Can you work these out from the drawing? Everything is in mm from the part's minimum corner. A direction names the side the tool comes from. Round coordinates to 2 decimals unless told otherwise and drop trailing zeros. Write each loop counter-clockwise with the first axis right and the second up, starting at its lowest first coordinate (ties: lowest second). Pieces come first, ordered by that corner, then holes. Notation, with made-up numbers: M 63.25,30 L 71.25,30 A15 ccw 71.25,35 Z; hole C -13.75,11 d9. An arc over 180 degrees is marked long. Answer in a Markdown table with one row per item. Add a question column.
(1) If I drill on probe 1 along Y at (x, z) = (10.5, 9.75); probe 2 along Z at (x, y) = (15, 16); probe 3 along Y at (x, z) = (10.5, 20), over which ranges is the centre line in solid material (lowest first)?
(2) Suppose I cut it at D-D, the plane y = 14.75. Write out the boundary of the cut face in (x, z).
(3) Suppose I cut it at A-A, the plane x = 10.5. Write out the boundary of the cut face in (y, z).
(4) For the marked faces 1 and 2, which set-ups out of +Z, -Z, +X, -X, +Y, -Y let a thin tool reach every point of the face, with its end or its side?
(5) Suppose I cut it at B-B, the plane y = 8.5. Write out the boundary of the cut face in (x, z), then the cut area to 3 significant figures.
(6) I'm going to push flat-ended pins straight in: pin 1 (12 mm diameter, centred on x = 9.5, y = 11, fed in from -Z); pin 2 (3 mm diameter, centred on x = 15, z = 4.5, fed in from +Y); pin 3 (2 mm diameter, centred on x = 4.5, z = 23, fed in from -Y); pin 4 (6 mm diameter, centred on y = 15, z = 6.5, fed in from +X). Where does each tip first touch, or does it pass through?
(7) Suppose I cut it at C-C, the plane z = 14.75. Write out the boundary of the cut face in (x, y), then the cut area to 3 significant figures.
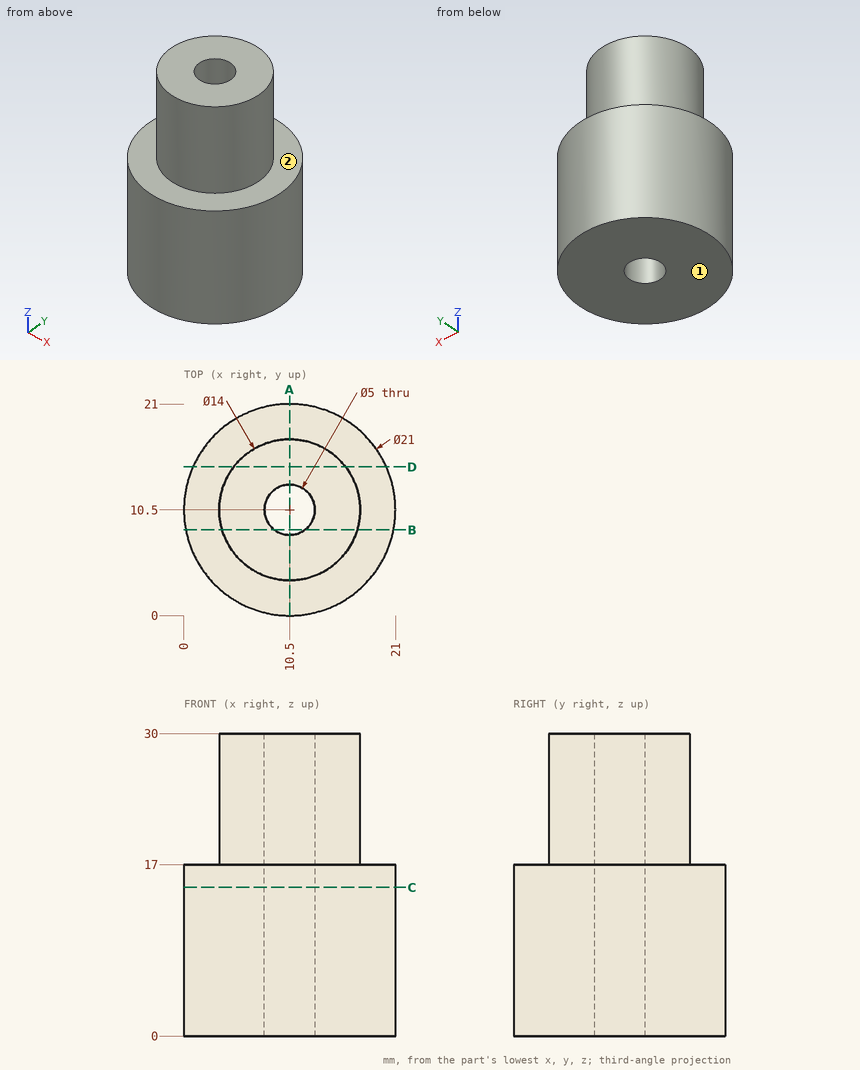
Calculated:
| question | item | result |
|---|---|---|
| 1 | probe 1 | 0 to 8, 13 to 21 |
| 1 | probe 2 | 0 to 17 |
| 1 | probe 3 | 3.5 to 8, 13 to 17.5 |
| 2 | outline | M 0.9,0 L 20.1,0 L 20.1,17 L 16.06,17 L 16.06,30 L 4.94,30 L 4.94,17 L 0.9,17 Z |
| 3 | outline | M 0,0 L 8,0 L 8,30 L 3.5,30 L 3.5,17 L 0,17 Z; M 13,0 L 21,0 L 21,17 L 17.5,17 L 17.5,30 L 13,30 Z |
| 4 | face 1 | -Z, +X, -X, +Y, -Y |
| 4 | face 2 | +Z |
| 5 | outline | M 0.19,0 L 9,0 L 9,30 L 3.79,30 L 3.79,17 L 0.19,17 Z; M 12,0 L 20.81,0 L 20.81,17 L 17.21,17 L 17.21,30 L 12,30 Z |
| 5 | area | 435 mm² |
| 6 | pin 1 | z = 0 |
| 6 | pin 2 | y = 20.56 |
| 6 | pin 3 | y = 5.6 |
| 6 | pin 4 | x = 20.89 |
| 7 | outline | C 10.5,10.5 d21; hole C 10.5,10.5 d5 |
| 7 | area | 327 mm² |
